```python
from build123d import *

# Parameters (mm, degrees)
ESTRUSIONE_ESTRUSIONE1_OUTLINE_W   = 10
ESTRUSIONE_ESTRUSIONE1_OUTLINE_H   = 8
ESTRUSIONE_ESTRUSIONE1_OUTLINE_W_2 = 12
ESTRUSIONE_ESTRUSIONE1_OUTLINE_H_2 = 22.6
ESTRUSIONE_ESTRUSIONE1_DEPTH       = 4
RACCORDO1_R                        = 1
RACCORDO3_R                        = 0.5
RACCORDO4_R                        = 0.3
SCHIZZO3_W                         = 31.69719665
SCHIZZO3_H                         = 4
ESTRUSIONE_ESTRUSIONE2_DEPTH       = 5


# Read off the part's stored shape, not the designer's step: Estrusione-Estrusione1
with BuildPart() as part:
    # Estrusione-Estrusione1 outline → Estrusione-Estrusione1 (new body)
    with BuildSketch(Plane.XY):
        with BuildLine():
            Line((-35.5, 26.1), (-39.5, 26.1))
            Line((-39.5, 26.1), (-39.5, 29.6))
            add(Edge.make_bspline(
                [(-39.5, 29.6), (-43.506938427, 25.593061573), (-43.493061573, 14.8), (-43.506938427, 4.006938427), (-39.5, 0)],
                knots=[0, 0, 0, 0, 0.5, 1, 1, 1, 1], degree=3))
            Line((-39.5, 0), (-39.5, 3.5))
            Line((-39.5, 3.5), (-35.5, 3.5))
            Line((-35.5, 3.5), (-35.5, 0))
            Line((-35.5, 0), (35.5, 0))
            Line((35.5, 0), (35.5, 3.5))
            Line((35.5, 3.5), (39.5, 3.5))
            Line((39.5, 3.5), (39.5, 0))
            add(Edge.make_bspline(
                [(39.5, 29.6), (43.506938427, 25.593061573), (43.493061573, 14.8), (43.506938427, 4.006938427), (39.5, 0)],
                knots=[0, 0, 0, 0, 0.5, 1, 1, 1, 1], degree=3))
            Line((39.5, 29.6), (39.5, 26.1))
            Line((39.5, 26.1), (35.5, 26.1))
            Line((35.5, 26.1), (35.5, 29.6))
            add(Edge.make_bspline(
                [(35.5, 29.6), (31.962623794, 26.062612753), (26.4060962, 25.659880805), (20.342579531, 28.112334068), (15.848598331, 29.600000017)],
                knots=[0, 0, 0, 0, 0.358970883, 0.890087037, 0.890087037, 0.890087037, 0.890087037], degree=3))
            Line((15.848598331, 29.600000017), (-15.848598331, 29.600000017))
            add(Edge.make_bspline(
                [(-35.5, 29.6), (-31.962623794, 26.062612753), (-26.4060962, 25.659880805), (-20.342579531, 28.112334068), (-15.848598331, 29.600000017)],
                knots=[0, 0, 0, 0, 0.358970883, 0.890087037, 0.890087037, 0.890087037, 0.890087037], degree=3))
            Line((-35.5, 29.6), (-35.5, 26.1))
        make_face()
        with Locations((-18, 6.6)):
            Rectangle(ESTRUSIONE_ESTRUSIONE1_OUTLINE_W, ESTRUSIONE_ESTRUSIONE1_OUTLINE_H, mode=Mode.SUBTRACT)
        with Locations((18, 6.6)):
            Rectangle(ESTRUSIONE_ESTRUSIONE1_OUTLINE_W, ESTRUSIONE_ESTRUSIONE1_OUTLINE_H, mode=Mode.SUBTRACT)
        with Locations((0, 13.3)):
            Rectangle(ESTRUSIONE_ESTRUSIONE1_OUTLINE_W_2, ESTRUSIONE_ESTRUSIONE1_OUTLINE_H_2, mode=Mode.SUBTRACT)
        Polygon((-25.868240888, 20.524038765), (-16.020163358, 22.260520542), (-15.15192247, 17.336481777), (-25, 15.6), align=None, mode=Mode.SUBTRACT)
        Polygon((16.020163358, 22.260520542), (25.868240888, 20.524038765), (25, 15.6), (15.15192247, 17.336481777), align=None, mode=Mode.SUBTRACT)
    extrude(amount=ESTRUSIONE_ESTRUSIONE1_DEPTH)

    # Raccordo1
    raccordo1_edges = [part.edges().sort_by_distance(p)[0] for p in [
        (16.020163358, 22.260520542, 2),
        (15.15192247, 17.336481777, 2),
        (25, 15.6, 2),
        (25.868240888, 20.524038765, 2),
        (-25.868240888, 20.524038765, 2),
        (-25, 15.6, 2),
        (-15.15192247, 17.336481777, 2),
        (-16.020163358, 22.260520542, 2),
    ]]
    fillet(raccordo1_edges, radius=RACCORDO1_R)

    # Raccordo3
    raccordo3_edges = [part.edges().sort_by_distance(p)[0] for p in [
        (13, 10.6, 2),
        (13, 2.6, 2),
        (23, 2.6, 2),
        (23, 10.6, 2),
        (-23, 10.6, 2),
        (-23, 2.6, 2),
        (-13, 2.6, 2),
        (-13, 10.6, 2),
    ]]
    fillet(raccordo3_edges, radius=RACCORDO3_R)

    # Raccordo4
    raccordo4_edges = [part.edges().sort_by_distance(p)[0] for p in [
        (-39.5, 0, 2),
        (39.5, 0, 2),
        (39.5, 29.6, 2),
        (35.5, 29.6, 2),
        (-39.5, 29.6, 2),
        (-35.5, 29.6, 2),
        (35.5, 0, 2),
        (-35.5, 0, 2),
    ]]
    fillet(raccordo4_edges, radius=RACCORDO4_R)

    # Schizzo3 → Estrusione-Estrusione2 (add)
    with BuildSketch(Plane(origin=(0, 29.6, 0), x_dir=(1, 0, 0), z_dir=(0, 1, 0))):
        with Locations((0, -2)):
            Rectangle(SCHIZZO3_W, SCHIZZO3_H)
    extrude(amount=ESTRUSIONE_ESTRUSIONE2_DEPTH)


solid = part.part
```
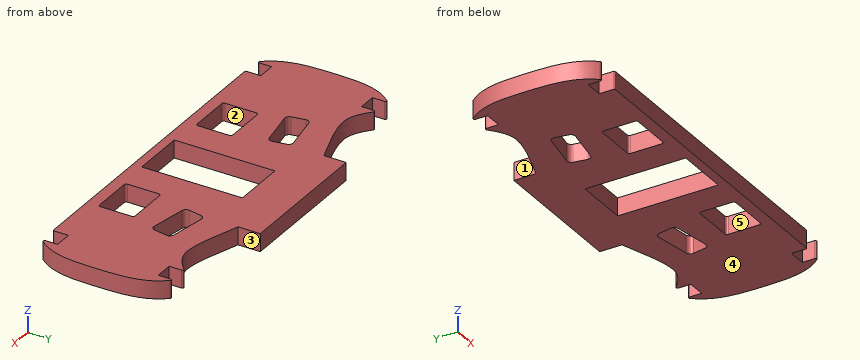
Verification items for the finished model (mm, model axes). Face numbers are marked on the shaded views. A direction names the side the tool comes from. Round coordinates to 2 decimals unless told otherwise and drop trailing zeros.
1) Draft check along X on the marked faces 1, 2 and 3. Enter one of: +X half, -X half, draft (parallel to the pull), parting line (faces both ways), or undercut.
Geometry says:
face 1: -X half
face 2: undercut
face 3: +X half
2) Depth check by flat-ended pin: pin 1 (2 mm diameter, centred on y = 6, z = 2, fed in from -X); pin 2 (0.8 mm diameter, centred on y = 27, z = 2, fed in from -X); pin 3 (8 mm diameter, centred on x = 18, y = 8, fed in from +Z); pin 4 (1.2 mm diameter, centred on y = 18.5, z = 3, fed in from -X). Enter the tip coordinate at first touch or a pass-through.
Geometry says:
pin 1: stops at x = -43.03
pin 2: stops at x = -41.69
pin 3: stops at z = 4
pin 4: stops at x = -43.47
3) Tool access check on the marked faces 4 and 5. Record the directions out of +Z, -Z, +X, -X, +Y, -Y that give a thin tool (end or side, any length) a straight path to the whole face; none if there is none.
Geometry says:
face 4: -Z, +X, -X, +Y, -Y
face 5: +Z, -Z
4) Cross-section at A-A, the plane x = -19. Give the number of separate pieces and of enclosed holes in the cut face, plus the area to 3 significant figures.
Geometry says:
separate pieces: 3
enclosed holes: 0
area: 61.8 mm2
5) Material ranges on line 1 (X direction, y = 9, z = 3); line 2 (X direction, y = 10.5, z = 3.8); line 3 (Y direction, x = 17.5, z = 3.6), recorded low to high.
Geometry says:
line 1: x = -43.31 to -23, -13 to -6, 6 to 13, 23 to 43.31
line 2: x = -43.42 to -22.8, -13.2 to -6, 6 to 13.2, 22.8 to 43.42
line 3: y = 0 to 2.6, 10.6 to 16.92, 22 to 29.04
